from build123d import *

# Parameters (mm, degrees)
BOSS_EXTRU_1_DEPTH      = 6
ESQUISSE2_R             = 1.25
ESQUISSE2_W             = 10
ESQUISSE2_H             = 10
ENL_V_MAT_EXTRU_1_DEPTH = 10
ESQUISSE4_W             = 20
ESQUISSE4_H             = 6
BOSS_EXTRU_2_DEPTH      = 6


with BuildPart() as part:
    # Esquisse1 → Boss.-Extru.1 (new body)
    with BuildSketch(Plane.XY):
        Polygon((-78, 0), (-78, 124.966679003), (0, 170), (0, 0), align=None)
    extrude(amount=BOSS_EXTRU_1_DEPTH)

    # Esquisse2 → Enlèv. mat.-Extru.1 (cut)
    with BuildSketch(Plane.XY.offset(6)):
        with Locations((-68, 126.121379542)):
            Circle(ESQUISSE2_R)
        with Locations((-50.679491924, 136.121379542)):
            Circle(ESQUISSE2_R)
        with Locations((-16.038475773, 156.121379542)):
            Circle(ESQUISSE2_R)
        with Locations((-33.358983849, 146.121379542)):
            Circle(ESQUISSE2_R)
        with Locations((-5, 5)):
            Rectangle(ESQUISSE2_W, ESQUISSE2_H)
    extrude(amount=-ENL_V_MAT_EXTRU_1_DEPTH, mode=Mode.SUBTRACT)

    # Esquisse4 → Boss.-Extru.2 (add)
    with BuildSketch(Plane.XZ):
        with Locations((-35, 3)):
            Rectangle(ESQUISSE4_W, ESQUISSE4_H)
    extrude(amount=BOSS_EXTRU_2_DEPTH)


solid = part.part
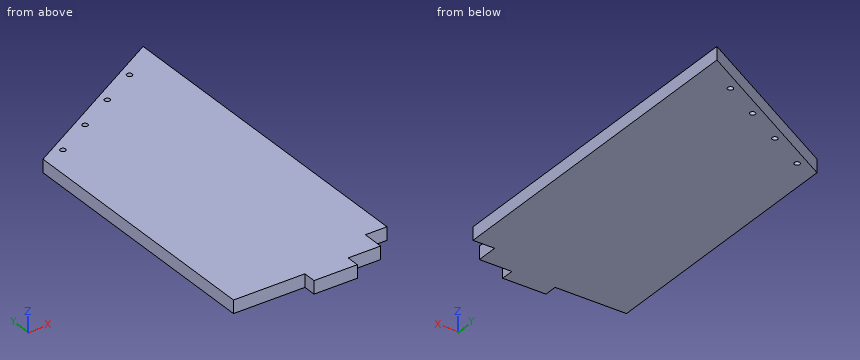
Source: CAD feature listing. Evaluate the final solid. Frame: model axes, mm. Round coordinates to 2 decimals unless told otherwise and drop trailing zeros. Loops run counter-clockwise (first coordinate to the right, second up) from the corner with the lowest first, then second, coordinate; pieces in that order, holes last. Notation, with made-up numbers: (10, 9.5) - (68, 9.5) arc R24 cw to (68, 27.5) - close; hole circle Ø9 at (-13, 37.25). An arc over 180 degrees is marked (long way). Write item = value, one per line. Start each with the question number.
(1) Section query A-A, the plane z = 5.1. Output: boundary loops of the cut face in (x, y), plus the area to 3 significant figures.
(2) Section query B-B, the plane x = -8. Output: boundary loops of the cut face in (y, z).
(3) Section query C-C, the plane x = -38. Output: boundary loops of the cut face in (y, z).
(4) Pin query (flat end, axial travel): pin 1 (3 mm diameter, centred on y = -3, z = 3.5, fed in from -X); pin 2 (1.5 mm diameter, centred on y = 82.5, z = 3, fed in from +X); pin 3 (1.8 mm diameter, centred on x = -19.5, z = 2.5, fed in from -Y). Return the tip coordinate at first contact, or that it passes through.
(5) Ray query, line 1 along X through (y, z) = (163.5, 4.6); line 2 along Y through (x, z) = (-60.5, 4.3); line 3 along Y through (x, z) = (-9, 3.05). Return the intervals inside material, ascending. Write a range as from..to.
Conclusion:
q1.outline = (-78, 0) - (-45, 0) - (-45, -6) - (-25, -6) - (-25, 0) - (-10, 0) - (-10, 10) - (0, 10) - (0, 170) - (-78, 124.97) - close; hole circle Ø2.5 at (-68, 126.12); hole circle Ø2.5 at (-50.68, 136.12); hole circle Ø2.5 at (-33.36, 146.12); hole circle Ø2.5 at (-16.04, 156.12)
q1.area = 11,500 mm2
q2.outline = (10, 0) - (165.38, 0) - (165.38, 6) - (10, 6) - close
q3.outline = (-6, 0) - (148.06, 0) - (148.06, 6) - (-6, 6) - close
q4.pin_1 = -45
q4.pin_2 = 0
q4.pin_3 = 0
q5.line_1 = -11.26..0
q5.line_2 = 0..135.07
q5.line_3 = 10..164.8
